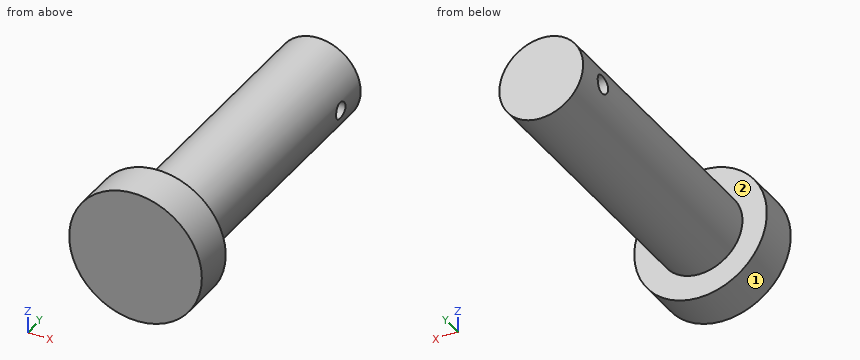
Solid Edge part; units mm, degrees
sketch "Sketch1" plane through (0, 0, 0) normal (0, -1, 0) x (1, 0, 0)
  circle A0 centre (0, 0) radius 12
extrude "Protrusion1" add sketch "Sketch1" along normal mid plane 80
sketch "Sketch2" plane through (0, -40, 0) normal (0, -1, 0) x (1, 0, 0)
  circle A0 centre (0, 0) radius 19
extrude "ExtrudedProtrusion_3" add sketch "Sketch2" along normal blind 12
sketch "Sketch3" plane through (0, 0, 0) normal (0, 0, 1) x (1, 0, 0)
  line L0 (0, 30.0534) -> (22, 30.0534)
  line L1 (22, 30.0534) -> (22, 27.7734)
  line L2 (-22, 27.3334) -> (22, 27.7734)
  line L3 (-22, 30.0534) -> (-22, 27.3334)
  line L4 (0, 30.0534) -> (-22, 30.0534)
revolve "RevolvedCutout1" cut sketch "Sketch3" angle 360 about axis through (0, 30.0534, 0) along (1, 0, 0)
properties material "Mild Steel"
CAD build for the part. Positions are in the model's coordinates, mm. Face numbers are marked on the shaded views. A direction names the side the tool comes from. Give positions to 0.01 mm unless a question says otherwise; leave off trailing zeros. Write each loop counter-clockwise with the first axis right and the second up, starting at its lowest first coordinate (ties: lowest second). Pieces come first, ordered by that corner, then holes. Notation, with made-up numbers: (-26, 5.5) - (26, 5.5) arc R7 ccw to (26, 13.5) - close; hole circle Ø2 at (72, 21). An arc over 180 degrees is marked (long way). Put each result on its own line as item: value.
(1) Tool access for the marked faces 1 and 2: list every direction of +Z, -Z, +X, -X, +Y, -Y with a clear straight run to the whole face (end or side of a thin tool).
Working result:
face 1: +Y, -Y
face 2: +Y
(2) Saw through at B-B (z = 10.5). List the corners of the cut face in (x, y).
Working result:
outline: (-15.84, -52) - (15.84, -52) - (15.84, -40) - (5.81, -40) - (5.81, 40) - (-5.81, 40) - (-5.81, -40) - (-15.84, -40) - close
(3) Saw through at A-A (x = 11). List the corners of the cut face in (y, z).
Working result:
outline: (-52, -15.49) - (-40, -15.49) - (-40, -4.8) - (40, -4.8) - (40, 4.8) - (-40, 4.8) - (-40, 15.49) - (-52, 15.49) - close; hole circle Ø4.78 at (30.05, 0)
(4) Wall check: L1, parallel to Y at x = -9.5, z = 11; L2, parallel to Z at x = 1, y = 30; L3, parallel to Y at x = 8.5, z = -2. Give the ranges that are in metal, low to high.
Working result:
L1: -52 to -40
L2: -11.96 to -2.49, 2.49 to 11.96
L3: -52 to 28.7, 31.41 to 40
(5) Drop flat-ended pins along their axis: pin 1 Ø2 at (y, z) = (-40, 2) entering from -X; pin 2 Ø5 at (x, y) = (-3.5, -4.5) entering from +Z; pin 3 Ø1.5 at (x, y) = (9, 4.5) entering from +Z. Give the stop position or say it passes through.
Working result:
pin 1: x = -18.97
pin 2: z = 11.96
pin 3: z = 8.71
(6) Saw through at D-D (x = -1). List the corners of the cut face in (y, z).
Working result:
outline: (-52, -18.97) - (-40, -18.97) - (-40, -11.96) - (40, -11.96) - (40, 11.96) - (-40, 11.96) - (-40, 18.97) - (-52, 18.97) - close; hole circle Ø5.02 at (30.05, 0)
(7) Saw through at C-C (y = 4.5). List the corners of the cut face in (x, z).
Working result:
outline: circle Ø24 at (0, 0)
